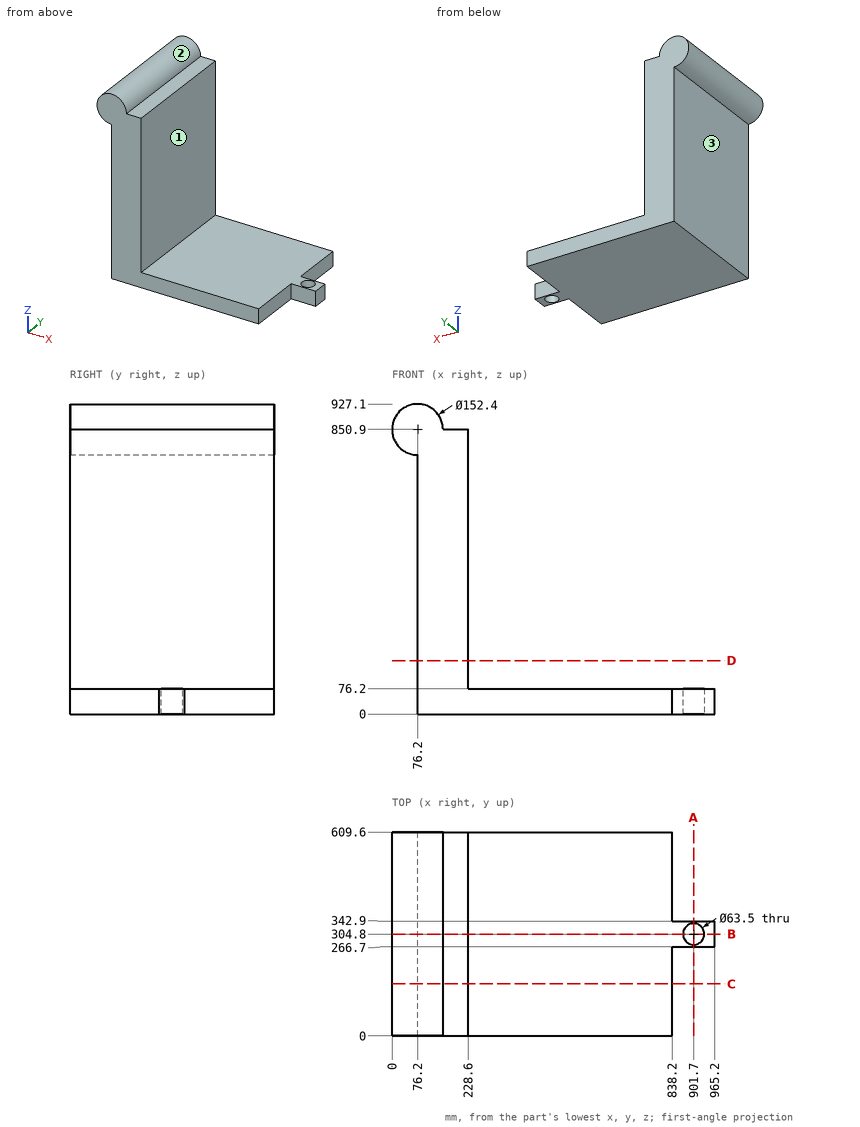
For this review, use the dimensioned drawing (mm, ordinates from the lowest corner) and the shaded views. A direction names the side the tool comes from. Round coordinates to 2 decimals unless told otherwise and drop trailing zeros. Write each loop counter-clockwise with the first axis right and the second up, starting at its lowest first coordinate (ties: lowest second). Pieces come first, ordered by that corner, then holes. Notation, with made-up numbers: (-13.75, 20.5) - (33.25, 20.5) arc R19 ccw to (33.25, 37.5) - close; hole circle Ø6 at (69, 62). An arc over 180 degrees is marked (long way). Answer as CSV lines item,"result". Start each with the question number.
(1) For pin 1 Ø6 at (y, z) = (435, 101.5) entering from +X; pin 2 Ø23 at (x, z) = (881, 37) entering from -Y; pin 3 Ø10 at (y, z) = (312.5, 637) entering from -X; pin 4 Ø12 at (x, y) = (847, 73.5) entering from -Z, all flat-tipped, find the tip position at first contact; note any pin that passes through.
(2) We need section B-B on y = 304.8. State the section outline as (x, z) points.
(3) For the marked faces 1, 2 and 3, list the 3-axis set-ups (+Z, -Z, +X, -X, +Y, -Y) from which the entire face can be reached by the end or side of a thin tool; tool diameter is ignored.
(4) We need section D-D on z = 160. State the section outline as (x, y) points, plus the area to 3 significant figures.
(5) To check wall thickness, follow line 1 (Y direction, x = 901, z = 24); line 2 (X direction, y = 304, z = 43); line 3 (Z direction, x = 618, y = 38). State the ranges of each line that lie inside material, in increasing order.
(6) We need section A-A on x = 901.7. State the section outline as (y, z) points, plus the area to 3 significant figures.
(7) We need section C-C on y = 156. State the section outline as (x, z) points.
Worked answers:
1,pin 1,"x = 228.6"
1,pin 2,"y = 266.7"
1,pin 3,"x = 76.2"
1,pin 4,"through"
2,outline,"(76.2, 0) - (869.95, 0) - (869.95, 76.2) - (228.6, 76.2) - (228.6, 850.9) - (152.4, 850.9) arc R76.2 ccw (long way) to (76.2, 774.7) - close; (933.45, 0) - (965.2, 0) - (965.2, 76.2) - (933.45, 76.2) - close"
3,face 1,"+Z, +X, +Y, -Y"
3,face 2,"+Y, -Y"
3,face 3,"-Z, -X, +Y, -Y"
4,outline,"(76.2, 0) - (228.6, 0) - (228.6, 609.6) - (76.2, 609.6) - close"
4,area,"92,900 mm²"
5,line 1,"266.7 to 273.06, 336.54 to 342.9"
5,line 2,"76.2 to 869.96, 933.44 to 965.2"
5,line 3,"0 to 76.2"
6,outline,"(266.7, 0) - (273.05, 0) - (273.05, 76.2) - (266.7, 76.2) - close; (336.55, 0) - (342.9, 0) - (342.9, 76.2) - (336.55, 76.2) - close"
6,area,"968 mm²"
7,outline,"(76.2, 0) - (838.2, 0) - (838.2, 76.2) - (228.6, 76.2) - (228.6, 850.9) - (152.4, 850.9) arc R76.2 ccw (long way) to (76.2, 774.7) - close"
